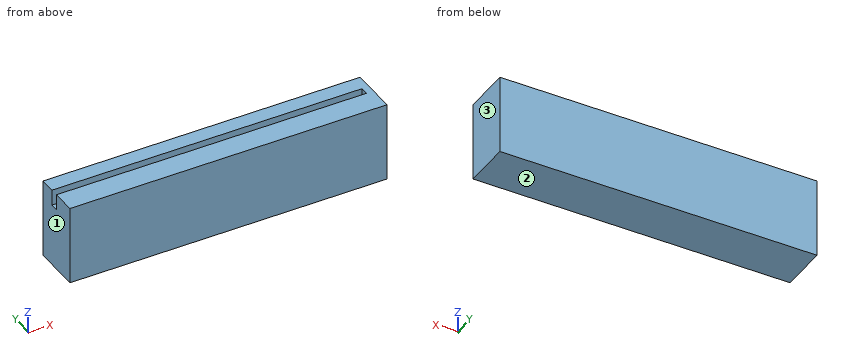
```python
from build123d import *

# Parameters (mm, degrees)
F0_W     = 101.6
F0_H     = 25.4
F1_DEPTH = 15.24
F2_W     = 99.3054434657
F2_H     = 2.54
F3_DEPTH = 5.08


# Not quite as in the source:
# - the program builds the solid bodies; features that only make, move or delete a surface that nothing else refers to are left out


with BuildPart() as f1:
    # F0 (on Front) → F1 (new body)
    with BuildSketch(Plane.XZ):
        with Locations((50.8, 12.7)):
            Rectangle(F0_W, F0_H)
    extrude(amount=F1_DEPTH)

    # F2 (on face) → F3 (cut)
    with BuildSketch(Plane.XY.offset(25.4)):
        with Locations((49.6527217329, -6.35)):
            Rectangle(F2_W, F2_H)
    extrude(amount=-F3_DEPTH, mode=Mode.SUBTRACT)


solid = f1.part
```
Source: CAD feature listing. Evaluate the final solid. Frame: model axes, mm. Face numbers are marked on the shaded views. Round coordinates to 2 decimals unless told otherwise and drop trailing zeros. Loops run counter-clockwise (first coordinate to the right, second up) from the corner with the lowest first, then second, coordinate; pieces in that order, holes last. Notation, with made-up numbers: (-16, 0) - (21, 0) arc R30 ccw to (21, 34) - close; hole circle Ø9 at (-30.75, 38). An arc over 180 degrees is marked (long way). Use CSV: the item, a comma, the result in double quotes.
Q1. Pin query (flat end, axial travel): pin 1 Ø2 at (x, y) = (66, -6.5) entering from +Z; pin 2 Ø0.8 at (y, z) = (-7, 22) entering from -X. Return the tip coordinate at first contact, or that it passes through.
Reported:
pin 1,"z = 20.32"
pin 2,"x = 99.31"
Q2. Ray query, line 1 along Y through (x, z) = (13, 23); line 2 along Z through (x, y) = (41, -7.5); line 3 along X through (y, z) = (-5.25, 21.75). Return the intervals inside material, ascending.
Reported:
line 1,"-15.24 to -7.62, -5.08 to 0"
line 2,"0 to 20.32"
line 3,"99.31 to 101.6"
Q3. Section query A-A, the plane x = 58. Output: boundary loops of the cut face in (y, z).
Reported:
outline,"(-15.24, 0) - (0, 0) - (0, 25.4) - (-5.08, 25.4) - (-5.08, 20.32) - (-7.62, 20.32) - (-7.62, 25.4) - (-15.24, 25.4) - close"
Q4. Section query B-B, the plane z = 23. Output: boundary loops of the cut face in (x, y), then the cut area to 3 significant figures.
Reported:
outline,"(0, -15.24) - (101.6, -15.24) - (101.6, 0) - (0, 0) - (0, -5.08) - (99.31, -5.08) - (99.31, -7.62) - (0, -7.62) - close"
area,"1,300 mm^2"
Q5. Mould query, pull axis X, two halves, no side actions, for the marked faces 1, 2 and 3. Classes: pulls with the +X half, pulls with the -X half, needs draft (parallel to the pull), parting line crosses it, or undercut.
Reported:
face 1,"pulls with the -X half"
face 2,"needs draft"
face 3,"pulls with the +X half"
